Autodesk Inventor part; units mm, degrees
ref_plane "YZ Plane" through (0, 0, 0) normal (1, 0, 0) x (0, 1, 0)
ref_plane "XZ Plane" through (0, 0, 0) normal (0, 1, 0) x (-1, 0, 0)
ref_plane "XY Plane" through (0, 0, 0) normal (0, 0, 1) x (1, 0, 0)
sketch "Sketch2" plane through (0, 0, 0) normal (0, 1, 0) x (-1, 0, 0)
  line L0 (-94, 28.5) -> (94, 28.5) construction
  line L1 (94, 28.5) -> (94, -28.5) construction
  line L2 (94, -28.5) -> (-94, -28.5) construction
  line L3 (-94, -28.5) -> (-94, 28.5) construction
  line L4 (-94, 28.5) -> (94, -28.5) construction
  line L5 (94, 28.5) -> (-94, -28.5) construction
  line L6 (78.6703, -31.5) -> (-78.6703, -31.5)
  line L7 (-97, -13.1703) -> (-97, 13.1703)
  line L8 (-78.6703, 31.5) -> (78.6703, 31.5)
  line L9 (97, 13.1703) -> (97, -13.1703)
  arc A0 (89.2832, -34.9615) -> (100.4615, -23.7832) centre (94, -28.5) ccw
  arc A1 (100.4615, 23.7832) -> (89.2832, 34.9615) centre (94, 28.5) ccw
  arc A2 (-89.2832, 34.9615) -> (-100.4615, 23.7832) centre (-94, 28.5) ccw
  arc A3 (-100.4615, -23.7832) -> (-89.2832, -34.9615) centre (-94, -28.5) ccw
  arc A4 (89.2832, -34.9615) -> (78.6703, -31.5) centre (78.6703, -49.5) ccw
  arc A5 (97, -13.1703) -> (100.4615, -23.7832) centre (115, -13.1703) ccw
  arc A6 (100.4615, 23.7832) -> (97, 13.1703) centre (115, 13.1703) ccw
  arc A7 (78.6703, 31.5) -> (89.2832, 34.9615) centre (78.6703, 49.5) ccw
  arc A8 (-89.2832, 34.9615) -> (-78.6703, 31.5) centre (-78.6703, 49.5) ccw
  arc A9 (-97, 13.1703) -> (-100.4615, 23.7832) centre (-115, 13.1703) ccw
  arc A10 (-100.4615, -23.7832) -> (-97, -13.1703) centre (-115, -13.1703) ccw
  arc A11 (-78.6703, -31.5) -> (-89.2832, -34.9615) centre (-78.6703, -49.5) ccw
  circle A12 centre (94, -28.5) radius 1.6
  circle A13 centre (94, 28.5) radius 1.6
  circle A14 centre (-94, -28.5) radius 1.6
  circle A15 centre (-94, 28.5) radius 1.6
  circle A16 centre (94, -28.5) radius 3 construction
  circle A17 centre (94, 28.5) radius 3 construction
  circle A18 centre (-94, 28.5) radius 3 construction
  circle A19 centre (-94, -28.5) radius 3 construction
  point P0 (0, 0)
  point P1 (86.5838, -31.5)
  point P2 (-86.5838, -31.5)
  point P3 (-97, -21.0838)
  point P4 (-97, 21.0838)
  point P5 (-86.5838, 31.5)
  point P6 (86.5838, 31.5)
  point P7 (97, 21.0838)
  point P8 (97, -21.0838)
  dimension "d6" = 3
  dimension "d7" = 3
  dimension "d8" = 3
  dimension "d9" = 3
  dimension "d10" = 8
  dimension "d11" = 18
  dimension "d14" = 3.2
  dimension "d15" = 63
  dimension "d16" = 194
  dimension "d17" = 6
extrude "Extrusion1" add sketch "Sketch2" along normal blind 4.5
sketch "Sketch4" plane through (0, 4.5, 0) normal (0, 1, 0) x (1, 0, 0)
  circle A0 centre (-13, 0) radius 10
  circle A1 centre (13, 0) radius 10
  circle A2 centre (-75, 0) radius 10
  circle A3 centre (-49, 0) radius 10
  circle A4 centre (49, 0) radius 10
  circle A5 centre (75, 0) radius 10
  circle A6 centre (-31, -16.75) radius 1.9
  circle A7 centre (0, -16.75) radius 1.9
  circle A8 centre (31, -16.75) radius 1.9
  circle A9 centre (0, 16.75) radius 1.9
  point P0 (0, 0)
  dimension "d23" = 26
  dimension "d24" = 13
  dimension "d25" = 20
  dimension "d26" = 36
  dimension "d27" = 26
  dimension "d28" = 36
  dimension "d29" = 26
  dimension "d32" = 31
  dimension "d33" = 31
  dimension "d34" = 16.75
  dimension "d35" = 16.75
  dimension "d36" = 3.8
extrude "Extrusion3" cut sketch "Sketch4" against normal through all
sketch "Sketch5" plane through (0, 4.5, 0) normal (0, 1, 0) x (1, 0, 0)
  line L0 (78.6703, 31.5) -> (-78.6703, 31.5)
  line L1 (-54.9, 31.5) -> (-45.1, 31.5)
  line L2 (-45.1, 31.5) -> (-45.1, 14.8)
  line L3 (-45.1, 14.8) -> (-54.9, 14.8)
  line L4 (-54.9, 14.8) -> (-54.9, 31.5)
  line L5 (48.725, 31.5) -> (56.275, 31.5)
  line L6 (56.275, 31.5) -> (56.275, 19)
  line L7 (56.275, 19) -> (48.725, 19)
  line L8 (48.725, 19) -> (48.725, 31.5)
  point P0 (0, 0)
  point P1 (-50, 31.5)
  point P2 (52.5, 31.5)
  dimension "d37" = 50
  dimension "d38" = 52.5
  dimension "d39" = 9.8
  dimension "d40" = 7.55
  dimension "d41" = 12.5
  dimension "d42" = 16.7
extrude "Extrusion4" cut sketch "Sketch5" against normal through all
equation "\"d7\" = d6"
equation "\"d8\" = d6"
equation "\"d9\" = d8"
equation "\"d27\" = d23"
equation "\"d28\" = d26"
equation "\"d29\" = d23"
equation "\"d33\" = d32"
properties part number "Top"
Source: CAD feature listing. Evaluate the final solid. Frame: model axes, mm. A direction names the side the tool comes from. Give positions to 0.01 mm unless a question says otherwise; leave off trailing zeros. Write each loop counter-clockwise with the first axis right and the second up, starting at its lowest first coordinate (ties: lowest second). Pieces come first, ordered by that corner, then holes.
1. Pull-direction query (Z, two-part tool) for faces 5 (the face through (1, 2, 31.5)), 6 (the face through (-54.9, 2, -23)), 7 (the face through (-0.247, 2.282, -18.634)); classes: +Z half, -Z half, draft (parallel to the pull), parting line (faces both ways), or undercut.
2. First-contact query: pin 1 (6 mm diameter, centred on x = 14, z = 13.5, fed in from -Y); pin 2 (2 mm diameter, centred on y = 3.5, z = 16, fed in from -X); pin 3 (1.3 mm diameter, centred on x = -67.5, y = 3, fed in from -Z). Flat tips, straight axial feed; report the tip coordinate or a pass-through.
3. Section query A-A (x = -13). Return the cut outline in (y, z).
4. Section query D-D (x = -49). Return the cut outline in (y, z).
5. Material intervals for line 1 along X through (y, z) = (2.4, -21) (3 decimals); line 2 along X through (y, z) = (1.95, -16.75); line 3 along Z through (x, y) = (75, 1.65), sorted ascending.
6. Section query C-C (z = 0). Return the cut outline in (x, y), then the cut area to 3 significant figures.
7. Section query B-B (z = -16.75). Return the cut outline in (x, y).
8. Access query for faces 1 (the face through (65, 2, 0)), 2 (the face through (-97.912, 2.218, -18.827)), 3 (the face through (-84.327, 2.218, 32.412)), 4 (the face through (56.275, 2, -25)). Directions: +Z, -Z, +X, -X, +Y, -Y. A direction counts if a zero-diameter tool reaches every point of the face in a straight line with its end or side. Return the directions, or none.
Output values:
1. face 5: +Z half
1. face 6: draft
1. face 7: undercut
2. pin 1: stops at y = 0
2. pin 2: stops at x = -97.41
2. pin 3: stops at z = -31.5
3. outline: (0, -31.5) - (4.5, -31.5) - (4.5, -10) - (0, -10) - close; (0, 10) - (4.5, 10) - (4.5, 31.5) - (0, 31.5) - close
4. outline: (0, -14.8) - (4.5, -14.8) - (4.5, -10) - (0, -10) - close; (0, 10) - (4.5, 10) - (4.5, 31.5) - (0, 31.5) - close
5. line 1: x = -98.792 to -54.9, -45.1 to 48.725, 56.275 to 98.792
5. line 2: x = -97.36 to -54.9, -45.1 to -1.9, 1.9 to 97.36
5. line 3: z = -31.5 to -10, 10 to 31.5
6. outline: (-97, 0) - (-85, 0) - (-85, 4.5) - (-97, 4.5) - close; (-65, 0) - (-59, 0) - (-59, 4.5) - (-65, 4.5) - close; (-39, 0) - (-23, 0) - (-23, 4.5) - (-39, 4.5) - close; (-3, 0) - (3, 0) - (3, 4.5) - (-3, 4.5) - close; (23, 0) - (39, 0) - (39, 4.5) - (23, 4.5) - close; (59, 0) - (65, 0) - (65, 4.5) - (59, 4.5) - close; (85, 0) - (97, 0) - (97, 4.5) - (85, 4.5) - close
6. area: 333 mm2
7. outline: (-97.36, 0) - (-54.9, 0) - (-54.9, 4.5) - (-97.36, 4.5) - close; (-45.1, 0) - (-1.9, 0) - (-1.9, 4.5) - (-45.1, 4.5) - close; (1.9, 0) - (97.36, 0) - (97.36, 4.5) - (1.9, 4.5) - close
8. face 1: +Y, -Y
8. face 2: -X, +Y, -Y
8. face 3: +Z, +Y, -Y
8. face 4: -Z, +Y, -Y
